Part model, mm, in its own coordinate system. A direction names the side the tool comes from. Give positions to 0.01 mm unless a question says otherwise; leave off trailing zeros. Write each loop counter-clockwise with the first axis right and the second up, starting at its lowest first coordinate (ties: lowest second). Pieces come first, ordered by that corner, then holes.
from build123d import *

# Parameters (mm, degrees)
SKETCH_1_R          = 14
EXTRUDE_1_DEPTH     = 30
SKETCH_2_R          = 5
EXTRUDE_2_DEPTH     = 9
SKETCH_2_3_R        = 5
CUT_EXTRUDE_1_DEPTH = 5


with BuildPart() as part:
    # Sketch 1 → Extrude 1 (new body)
    with BuildSketch(Plane.XY):
        Circle(SKETCH_1_R)
    extrude(amount=EXTRUDE_1_DEPTH)

    # Sketch 2 → Extrude 2 (add, symmetric)
    with BuildSketch(Plane(origin=(0, 0, 0), x_dir=(1, 0, 0), z_dir=(0, 1, 0))):
        with BuildLine():
            Line((10, 15), (10, 0))
            Line((10, 0), (-10, 0))
            Line((-10, 0), (-10, 15))
            ThreePointArc((-10, 15), (0, 25), (10, 15))
        make_face()
        with Locations(Location((0, 15, 0), (0, 0, 270))):
            Circle(SKETCH_2_R, mode=Mode.SUBTRACT)
    extrude(amount=EXTRUDE_2_DEPTH, both=True)

    # Sketch 2_3 → Cut-Extrude 1 (cut, symmetric)
    with BuildSketch(Plane(origin=(0, 0, 0), x_dir=(1, 0, 0), z_dir=(0, 1, 0))):
        with BuildLine():
            Line((10, 15), (10, 0))
            Line((10, 0), (-10, 0))
            Line((-10, 0), (-10, 15))
            ThreePointArc((-10, 15), (0, 25), (10, 15))
        make_face()
        with Locations(Location((0, 15, 0), (0, 0, 270))):
            Circle(SKETCH_2_3_R, mode=Mode.SUBTRACT)
    extrude(amount=CUT_EXTRUDE_1_DEPTH, both=True, mode=Mode.SUBTRACT)


solid = part.part
1) Mould opens along Y. For faces 4 (the flat face through (2, -5, -10)), 5 (the flat face through (2, 5, -10)), 6 (the flat face through (2, 9, -10)), 7 (the flat face through (2, -9, -10)) say: +Y half, -Y half, draft (parallel to the pull), parting line (faces both ways), or undercut.
Check result:
face 4: undercut
face 5: undercut
face 6: +Y half
face 7: -Y half
2) Saw through at B-B (y = 6). Write the cut outline in (x, z), and give its area (3 significant figures).
Check result:
outline: (-12.65, 0) - (-10, 0) - (-10, -15) arc R10 ccw to (10, -15) - (10, 0) - (12.65, 0) - (12.65, 30) - (-12.65, 30) - close; hole circle Ø10 at (0, -15)
area: 1,140 mm2
3) Drill centre lines: L1, parallel to Y at x = -0.75, z = -7.5; L2, parallel to X at y = -7.9, z = -15; L3, parallel to Z at x = -11, y = -6.25. Where is each one in solid material? Low to high.
Check result:
L1: y = -9 to -5, 5 to 9
L2: x = -10 to -5, 5 to 10
L3: z = 0 to 30
4) Saw through at D-D (z = 3). Write the cut outline in (x, y).
Check result:
outline: circle Ø28 at (0, 0)
5) Saw through at A-A (x = 0). Write the cut outline in (y, z), and give its area (3 significant figures).
Check result:
outline: (-14, 0) - (-9, 0) - (-9, -10) - (-5, -10) - (-5, 0) - (5, 0) - (5, -10) - (9, -10) - (9, 0) - (14, 0) - (14, 30) - (-14, 30) - close; (-9, -25) - (-5, -25) - (-5, -20) - (-9, -20) - close; (5, -25) - (9, -25) - (9, -20) - (5, -20) - close
area: 960 mm2
6) 3-axis set-ups, long thin cutter, end or side, ignore diameter. For faces 1 (the cylindrical face through (0, -7, -25)), 2 (the flat face through (10, -7, -8)), 3 (the flat face through (-10, -7, -7)): which of +Z, -Z, +X, -X, +Y, -Y reach the whole face in a straight line?
Check result:
face 1: -Z, +Y, -Y
face 2: -Z, +X, +Y, -Y
face 3: -Z, -X, +Y, -Y
7) Saw through at C-C (z = -11.5). Write the cut outline in (x, y).
Check result:
outline: (-10, -9) - (-3.57, -9) - (-3.57, -5) - (-10, -5) - close; (-10, 5) - (-3.57, 5) - (-3.57, 9) - (-10, 9) - close; (3.57, -9) - (10, -9) - (10, -5) - (3.57, -5) - close; (3.57, 5) - (10, 5) - (10, 9) - (3.57, 9) - close
8) Flat gauge pins, fed straight in: P1, Ø4.5, axis at y = -8, z = -6.5, coming from the -X side; P2, Ø4.5, axis at y = 7, z = -6.5, coming from the +X side; P3, Ø1.5, axis at y = -9.5, z = -0.5, coming from the -X side; P4, Ø6, axis at x = 0, z = -15, coming from the -Y side. Where does each tip first touch, or does it go through?
Check result:
P1: stops at x = -10
P2: stops at x = 10
P3: stops at x = -10.77
P4: passes through
